Work out the finished part from the listing and answer in its coordinate system (mm). A direction names the side the tool comes from. Give positions to 0.01 mm unless a question says otherwise; leave off trailing zeros. Write each loop counter-clockwise with the first axis right and the second up, starting at its lowest first coordinate (ties: lowest second). Pieces come first, ordered by that corner, then holes.
1) Given pin 1 Ø1 at (x, z) = (-20, 9) entering from -Y; pin 2 Ø5.5 at (x, z) = (2.5, 32) entering from +Y; pin 3 Ø2 at (x, z) = (-16, 17) entering from -Y, each flat-ended and moving along its own axis, determine where each tip first touches the part or whether it passes through.
2) Find section B-B (y = -20.5). Determine the outline of the cut face in (x, z).
3) Find section D-D (x = 12.5). Determine the outline of the cut face in (y, z) (3 decimals), plus the area to 3 significant figures.
4) Straight lines are drawn through the part: probe 1 along Z at (x, y) = (-13, -35); probe 2 along Z at (x, y) = (-22, 11); probe 3 along Y at (x, z) = (23, 17). For each, find the intervals that lie inside material, in ascending order.
5) Determine the mould class of faces 3 (the face through (-1, 1, 0)), 4 (the face through (19.174, 32.924, 12.522)), 5 (the face through (-24.21, -13.55, 19.09)) for opening direction X: pulls with the +X half, pulls with the -X half, needs draft (parallel to the pull), parting line crosses it, or undercut.
6) A tool of negligible diameter and unlimited length cuts with its end or side. For faces 1 (the face through (-4.837, 7.593, 37.64)), 2 (the face through (33.067, 18.926, 12.522)), from which of +Z, -Z, +X, -X, +Y, -Y can it reach the whole face along a straight path? Write none if from no direction.
7) Find section C-C (z = 5). Determine the outline of the cut face in (x, y), plus the area to 3 significant figures.
8) Find section A-A (z = 24). Determine the outline of the cut face in (x, y).
```python
from build123d import *

# Parameters (mm, degrees)
F1_DEPTH = 25.4
F3_DEPTH = 12.80478
F5_DEPTH = 50.8


with BuildPart() as f1:
    # F0 (on Top) → F1 (new body)
    with BuildSketch(Plane.XY):
        Polygon((38.1, -10.208864), (38.1, 10.208864), (27.891136, 27.891136), (10.208864, 38.1), (-10.208864, 38.1), (-27.891136, 27.891136), (-38.1, 10.208864), (-38.1, -10.208864), (-27.891136, -27.891136), (-10.208864, -38.1), (10.208864, -38.1), (27.891136, -27.891136), align=None)
    extrude(amount=F1_DEPTH)

    # F2 (on face) → F3 (cut)
    with BuildSketch(Plane.XY.offset(25.4)):
        Polygon((18.787623, -22.776135), (29.032371, -5.37108), (25.692551, 14.547162), (10.3309, 27.658626), (-9.864694, 27.828311), (-25.444488, 14.97682), (-29.118523, -4.882491), (-19.167678, -22.457231), (-0.248063, -29.523983), align=None)
    extrude(amount=-F3_DEPTH, mode=Mode.SUBTRACT)

    # F4 (on face) → F5 (join)
    with BuildSketch(Plane.XY.offset(12.59522)):
        Polygon((-9.541287, 14.97682), (0, 0), (9.541287, 14.97682), align=None)
    extrude(amount=F5_DEPTH)


solid = f1.part
```
Results:
1. pin 1: stops at y = -32.74
1. pin 2: stops at y = 14.98
1. pin 3: stops at y = -35.33
2. outline: (-32.16, 0) - (32.16, 0) - (32.16, 25.4) - (20.13, 25.4) - (20.13, 12.6) - (-20.28, 12.6) - (-20.28, 25.4) - (-32.16, 25.4) - close
3. outline: (-36.777, 0) - (36.777, 0) - (36.777, 25.4) - (25.807, 25.4) - (25.807, 12.595) - (-25.005, 12.595) - (-25.005, 25.4) - (-36.777, 25.4) - close
3. area: 1,220 mm2
4. probe 1: z = 0 to 25.4
4. probe 2: z = 0 to 12.6
4. probe 3: y = -30.72 to -15.62, 16.85 to 30.72
5. face 3: needs draft
5. face 4: pulls with the +X half
5. face 5: undercut
6. face 1: +Z
6. face 2: +Z, -Z, +X, +Y
7. outline: (-38.1, -10.21) - (-27.89, -27.89) - (-10.21, -38.1) - (10.21, -38.1) - (27.89, -27.89) - (38.1, -10.21) - (38.1, 10.21) - (27.89, 27.89) - (10.21, 38.1) - (-10.21, 38.1) - (-27.89, 27.89) - (-38.1, 10.21) - close
7. area: 4,670 mm2
8. outline: (-38.1, -10.21) - (-27.89, -27.89) - (-10.21, -38.1) - (10.21, -38.1) - (27.89, -27.89) - (38.1, -10.21) - (38.1, 10.21) - (27.89, 27.89) - (10.21, 38.1) - (-10.21, 38.1) - (-27.89, 27.89) - (-38.1, 10.21) - close; (-9.54, 14.98) - (0, 0) - (9.54, 14.98) - close; hole (-29.12, -4.88) - (-19.17, -22.46) - (-0.25, -29.52) - (18.79, -22.78) - (29.03, -5.37) - (25.69, 14.55) - (10.33, 27.66) - (-9.86, 27.83) - (-25.44, 14.98) - close
